```python
from build123d import *

# Parameters (mm, degrees)
CIRPATTERN1_COUNT = 6


with BuildPart() as part:
    # chamberNozzle → Revolve1 (revolve)
    with BuildSketch(Plane.XY, mode=Mode.PRIVATE) as revolve1_sk:
        with BuildLine():
            Line((0, 38.1), (110.897045256, 38.1))
            ThreePointArc((110.897045256, 38.1), (114.184047129, 37.667257994), (117.247045256, 36.398522628))
            Line((117.247045256, 36.398522628), (153.648338424, 15.382226219))
            ThreePointArc((153.648338424, 15.382226219), (157.542961832, 14.060179716), (161.647049978, 14.329175865))
            Line((161.647049978, 14.329175865), (210.545228126, 27.431403211))
            Line((210.545228126, 27.431403211), (210.545228126, 78.231403211))
            Line((210.545228126, 78.231403211), (161.647049978, 65.129175865))
            ThreePointArc((161.647049978, 65.129175865), (157.542961832, 64.860179716), (153.648338424, 66.182226219))
            Line((153.648338424, 66.182226219), (117.247045256, 87.198522628))
            ThreePointArc((117.247045256, 87.198522628), (114.184047129, 88.467257994), (110.897045256, 88.9))
            Line((110.897045256, 88.9), (0, 88.9))
            Line((0, 88.9), (0, 55.88))
            Line((0, 55.88), (5.08, 55.88))
            Line((5.08, 55.88), (5.08, 45.72))
            Line((5.08, 45.72), (0, 45.72))
            Line((0, 45.72), (0, 38.1))
        make_face()
    revolve(revolve1_sk.sketch.rotate(Axis((0, 0, 0), (1, 0, 0)), 90), axis=Axis((0, 0, 0), (1, 0, 0)))

    # Sketch3 → 1/2 (0.5) Diameter Hole1 (revolve, cut)
    with BuildSketch(Plane(origin=(0, 0, -72.39), x_dir=(0, 0, 1), z_dir=(0, 1, 0))):
        Polygon((0, 0), (0, 16.515464931), (6.35, 12.7), (6.35, 0.635), (6.985, 0), align=None)
    f_1_2_0_5_diameter_hole1 = revolve(axis=Axis((-6.35, 0, -72.39), (1, 0, 0)), mode=Mode.SUBTRACT)

    # CirPattern1: 1/2 (0.5) Diameter Hole1 ×6 about axis
    cirpattern1_axis = Axis((0, 0, 0), (1, 0, 0))
    for i in range(1, CIRPATTERN1_COUNT):
        add(f_1_2_0_5_diameter_hole1.rotate(cirpattern1_axis, i * 360 / CIRPATTERN1_COUNT), mode=Mode.SUBTRACT)


solid = part.part
```
Input: part model. Units: mm. Frame: model coordinates. A direction names the side the tool comes from. Round coordinates to 2 decimals unless told otherwise and drop trailing zeros. Write each loop counter-clockwise with the first axis right and the second up, starting at its lowest first coordinate (ties: lowest second). Pieces come first, ordered by that corner, then holes. Notation, with made-up numbers: (2.5, 5) -> (28.5, 5) arc R19 ccw to (28.5, 24) -> close; hole circle Ø11 at (89.5, 57). An arc over 180 degrees is marked (long way). Answer as CSV lines item,"result".
1. Ray query, L1, parallel to Y at x = 128, z = -26.5; L2, parallel to Z at x = 186, y = 16; L3, parallel to Y at x = 22, z = 16.5. Return the intervals inside material, ascending. Write a range as [from, to].
Geometry says:
L1,"y = [-76.53, -14.46], [14.46, 76.53]"
L2,"z = [-69.85, -13.38], [13.38, 69.85]"
L3,"y = [-87.36, -34.34], [34.34, 87.36]"
2. Contact query for flat-ended pins moving along their axis: P1, Ø7.5, axis at y = -62.69, z = -36.2, coming from the -X side; P2, Ø8, axis at x = 83.5, z = 33.5, coming from the -Y side; P3, Ø12, axis at x = 121.5, z = 41.5, coming from the -Y side; P4, Ø1, axis at y = -32, z = -61.5, coming from the -X side. Output: stop coordinate, or through.
Geometry says:
P1,"stops at x = 14.26"
P2,"stops at y = -83.86"
P3,"stops at y = -78.87"
P4,"stops at x = 0"
3. Section B-B (x = 149.5). Return the cut outline in (y, z).
Geometry says:
outline,"circle Ø137.15 at (0, 0); hole circle Ø35.55 at (0, 0)"
4. Reachability of faces 3 (the flat face through (0, -37, -10)), 4 (the cylindrical face through (56.225, 37.194, -8.259)) from +Z, -Z, +X, -X, +Y, -Y: full face, straight path, thin tool, end or side. Return the list, or none.
Geometry says:
face 3,"+Z, -Z, -X, +Y, -Y"
face 4,"-X"
5. Mould query, pull axis Y, two halves, no side actions, for faces 1 (the flat face through (0, 58, -1)), 2 (the conical face through (15.853, 63.621, -36.788)). Classes: +Y half, -Y half, draft (parallel to the pull), parting line (faces both ways), or undercut.
Geometry says:
face 1,"draft"
face 2,"undercut"
